Autodesk Fusion 360 part; units mm, degrees
sketch "Sketch1" plane through (0, 0, 0) normal (0, 0, 1) x (1, 0, 0)
  line L0 (50, 20) -> (-50, 20)
  line L1 (-50, 20) -> (-50, -20)
  line L2 (-50, -20) -> (50, -20)
  line L3 (50, -20) -> (50, 20)
  line L4 (50, 20) -> (-50, -20) construction
  line L5 (-50, 20) -> (50, -20) construction
  line L6 (35.75, -1) -> (-35.75, -1)
  line L7 (-35.75, -1) -> (-35.75, -19)
  line L8 (-35.75, -19) -> (35.75, -19)
  line L9 (35.75, -19) -> (35.75, -1)
  line L10 (35.75, -1) -> (-35.75, -19) construction
  line L11 (-35.75, -1) -> (35.75, -19) construction
  line L12 (-29.75, -4) -> (-29.75, -16)
  line L13 (29.75, -16) -> (29.75, -4)
  line L14 (29.75, -4) -> (-29.75, -16) construction
  line L15 (-29.75, -4) -> (29.75, -16) construction
  line L16 (-6.75, -16) -> (-6.75, -4)
  line L17 (6.75, -4) -> (6.75, -16)
  line L18 (6.75, -16) -> (-6.75, -4) construction
  line L19 (-6.75, -16) -> (6.75, -4) construction
  line L20 (29.75, -4) -> (6.75, -4)
  line L21 (-6.75, -4) -> (-29.75, -4)
  line L22 (-29.75, -16) -> (-6.75, -16)
  line L23 (6.75, -16) -> (29.75, -16)
  circle A0 centre (-32.25, -10) radius 1.5
  circle A1 centre (32.25, -10) radius 1.5
  circle A2 centre (-4.25, -10) radius 1.5
  circle A3 centre (4.25, -10) radius 1.5
  line L24 (0, -1) -> (0, -19)
  line L25 (5, 0) -> (-5, 0)
  line L26 (-5, 0) -> (-5, -7)
  line L27 (-5, -7) -> (5, -7)
  line L28 (5, -7) -> (5, 0)
  line L29 (5, 0) -> (-5, -7) construction
  line L30 (-5, 0) -> (5, -7) construction
  point P0 (0, -10)
  point P1 (0, -10)
  point P2 (0, -10)
  point P3 (-32.25, -10)
  point P4 (32.25, -10)
  point P5 (-4.25, -10)
  point P6 (4.25, -10)
  point P7 (0, -3.5)
  dimension "d1" = 100
  dimension "d2" = 40
  dimension "d3" = 71.5
  dimension "d4" = 18
  dimension "d5" = 1
  dimension "d6" = 59.5
  dimension "d7" = 12
  dimension "d8" = 13.5
  dimension "d9" = 12
  dimension "d10" = 3.5
  dimension "d11" = 3
  dimension "d12" = 3.5
  dimension "d13" = 3
  dimension "d14" = 2.5
  dimension "d15" = 2.5
  dimension "d16" = 3
  dimension "d17" = 3
  dimension "d44" = 10
  dimension "d45" = 7
extrude "Extrude1" add sketch "Sketch1" along normal blind 3 contours L0 L1 L2 L3 | L6 L25 L26 L28 | L6 L24 L26 L27 | L6 L7 L8 L24 L26 L27 makes body 1
extrude "Extrude2" add sketch "Sketch1" along normal blind 6 and the other way blind -3 separate body contours L6 L8 L9 L24 L27 L28 | L6 L24 L27 L28 makes body 2
move_face "OffsetFaces1" offset 1 3 faces at (0, -7, 5) (23.8333, -1, 4) (35.75, -13, 5) on bodies 2
move_face "OffsetFaces2" offset 1 1 faces at (11.5833, -19, 5) on bodies 2
sketch "Sketch2" plane through (0, 0, 0) normal (0, 0, 1) x (1, 0, 0)
  line L0 (-50, 20) -> (-50, -20)
  line L1 (50, 20) -> (-50, 20)
  line L2 (50, -20) -> (50, 20)
  circle A0 centre (-30, 10) radius 2.5
  circle A1 centre (30, 10) radius 2.5
  circle A2 centre (-30, 10) radius 5
  circle A3 centre (30, 10) radius 5
  circle A4 centre (0, 10) radius 5
  circle A5 centre (0, 10) radius 2.5
  point P0 (-30, 10)
  point P1 (30, 10)
  dimension "d31" = 20
  dimension "d32" = 10
  dimension "d33" = 20
  dimension "d34" = 5
  dimension "d35" = 5
  dimension "d36" = 10
  dimension "d37" = 10
  dimension "d48" = 10
  dimension "d49" = 5
extrude "Extrude3" cut sketch "Sketch2" along normal blind 3 contours A0 | A1 bodies 1
extrude "Extrude4" cut sketch "Sketch2" along normal blind 3 and the other way blind -2 contours A2 | A3 bodies 1
combine "Combine1" operation add target body 2 tool bodies 1
extrude "Extrude5" cut sketch "Sketch1" along normal blind 6 contours L6 L24 L27 L28 | L6 L25 L26 L28 | L6 L24 L26 L27 bodies 2
Geometry: final body of the model. Coordinates: model frame, mm. A direction names the side the tool comes from. Coordinates: 2 decimals unless noted, no trailing zeros. Order: outer loops, then holes, each group sorted by start corner. A loop starts at its lowest first (then second) coordinate and runs counter-clockwise, first axis right, second up. Notation, with made-up numbers: M -35,81.25 L -14,81.25 A20 cw -14,104.25 Z; hole C -19,-35.75 d7. An arc over 180 degrees is marked long. Answer in a Markdown table with one row per item. Add a question column.
Q1. Section query A-A on x = -8. Return the cut outline in (y, z).
Q2. Contact query for flat-ended pins moving along their axis: P1, Ø6, axis at x = 30, y = 10, coming from the +Z side; P2, Ø3, axis at x = -33.5, y = 13.5, coming from the +Z side; P3, Ø0.9, axis at y = -10.5, z = 5, coming from the +X side. Output: stop coordinate, or through.
Q3. Reachability of faces 1 (the flat face through (32, 8, 2)), 2 (the flat face through (0, 0, 1)), 3 (the flat face through (-1, -13, 4)) from +Z, -Z, +X, -X, +Y, -Y: full face, straight path, thin tool, end or side. Return the list, or none.
Q4. Line query: L1, parallel to X at y = -10, z = 4.7; L2, parallel to Y at x = -4.25, z = 0.7; L3, parallel to Y at x = 30, z = 2.45. Output: solid intervals per line, ascending.
Q5. Section query B-B on y = -15. Return the cut outline in (x, z).
Q6. Section query C-C on z = 4.4. Return the cut outline in (x, y).
Q7. Section query D-D on y = 10. Return the cut outline in (x, z), and give its area (3 significant figures).
Q8. Mould query, pull axis Y, two halves, no side actions, for faces 4 (the flat face through (-18, -16, 1)), 5 (the flat face through (21, 0, 4)), 6 (the flat face through (-1, 5, 0)), 7 (the cylindrical face through (25.005, 9.78, 2.493)). Classes: released by +Y, released by -Y, zero draft, split by the parting line, or undercut.
Completed:
| question | item | result |
|---|---|---|
| 1 | outline | M -20,0 L -16,0 L -16,3 L -20,3 Z; M -4,0 L 20,0 L 20,3 L -4,3 Z |
| 2 | P1 | stops at z = 2 |
| 2 | P2 | stops at z = 3 |
| 2 | P3 | stops at x = 36.75 |
| 3 | face 1 | +Z |
| 3 | face 2 | +Z, -Z |
| 3 | face 3 | +Z, -X, +Y, -Y |
| 4 | L1 | x = -1 to 2.75, 5.75 to 6.75, 29.75 to 30.75, 33.75 to 36.75 |
| 4 | L2 | y = -20 to -11.5, -8.5 to -7, 0 to 20 |
| 4 | L3 | y = -20 to -19, -1 to 5, 15 to 20 |
| 5 | outline | M -50,0 L -29.75,0 L -29.75,3 L -50,3 Z; M -6.75,0 L 0,0 L 0,3 L 6.75,3 L 6.75,6 L -1,6 L -1,3 L -6.75,3 Z; M 29.75,3 L 35.75,3 L 35.75,0 L 50,0 L 50,3 L 36.75,3 L 36.75,6 L 29.75,6 Z |
| 6 | outline | M -1,-20 L 36.75,-20 L 36.75,0 L 5,0 L 5,-7 L -1,-7 Z; hole C 4.25,-10 d3; hole M 6.75,-16 L 29.75,-16 L 29.75,-4 L 6.75,-4 Z; hole C 32.25,-10 d3 |
| 7 | outline | M -50,0 L -32.5,0 L -32.5,2 L -35,2 L -35,3 L -50,3 Z; M -27.5,0 L 27.5,0 L 27.5,2 L 25,2 L 25,3 L -25,3 L -25,2 L -27.5,2 Z; M 32.5,0 L 50,0 L 50,3 L 35,3 L 35,2 L 32.5,2 Z |
| 7 | area | 260 mm2 |
| 8 | face 4 | undercut |
| 8 | face 5 | released by +Y |
| 8 | face 6 | zero draft |
| 8 | face 7 | undercut |
